from build123d import *

# Parameters (mm, degrees)
F0_W     = 38.1
F0_H     = 762
F0_W_2   = 63.5
F0_H_2   = 57.15
F0_W_3   = 152.4
F0_H_3   = 152.4
F1_DEPTH = 19.05


with BuildPart() as f1:
    # F0 (on Top) → F1 (new body)
    with BuildSketch(Plane.XY):
        Polygon((-669.859934, 405.539142), (-669.859934, -508.860858), (244.540066, -508.860858), (244.540066, 405.539142), (92.140066, 862.739142), (-517.459934, 862.739142), align=None)
        with Locations((-612.709934, -89.760858)):
            Rectangle(F0_W, F0_H, mode=Mode.SUBTRACT)
        with Locations((187.390066, -89.760858)):
            Rectangle(F0_W, F0_H, mode=Mode.SUBTRACT)
        with Locations((-600.009934, 376.964142)):
            Rectangle(F0_W_2, F0_H_2, mode=Mode.SUBTRACT)
        with Locations((-212.659934, 634.139142)):
            Rectangle(F0_W_3, F0_H_3, mode=Mode.SUBTRACT)
        with Locations((174.690066, 376.964142)):
            Rectangle(F0_W_2, F0_H_2, mode=Mode.SUBTRACT)
    extrude(amount=F1_DEPTH)


solid = f1.part
Check sheet for the modelled part. Datum: model origin and axes. Units: mm. Round coordinates to 2 decimals unless told otherwise and drop trailing zeros. Write each loop counter-clockwise with the first axis right and the second up, starting at its lowest first coordinate (ties: lowest second). Pieces come first, ordered by that corner, then holes. Notation, with made-up numbers: (67.5, 18.5) -> (109.5, 18.5) arc R12 cw to (109.5, 29.5) -> close; hole circle Ø6 at (85, 57.5). An arc over 180 degrees is marked (long way). Answer as CSV lines item,"result". Start each with the question number.
1) Material ranges on line 1 (X direction, y = -289.5, z = 4.25); line 2 (X direction, y = 357, z = 2); line 3 (Y direction, x = -166.5, z = 9), recorded low to high. Write a range as from..to.
2) Section check B-B on z = 7. Enter the section's corners in (x, y), and give its area (3 significant figures).
3) Section check D-D on y = 509. Enter the section's corners in (x, z), and give its area (3 significant figures).
4) Section check C-C on x = -197. Enter the section's corners in (y, z), and give its area (3 significant figures).
5) Go/stop test with a flat-tipped pin: P1, Ø5.5, axis at y = 670, z = 11.5, coming from the +X side. Record where the tip stops, or that it passes through.
6) Section check A-A on y = 29.5. Enter the section's corners in (x, z).
Found:
1,line 1,"x = -669.86..-631.76, -593.66..168.34, 206.44..244.54"
1,line 2,"x = -669.86..-631.76, -568.26..142.94, 206.44..244.54"
1,line 3,"y = -508.86..557.94, 710.34..862.74"
2,outline,"(-669.86, -508.86) -> (244.54, -508.86) -> (244.54, 405.54) -> (92.14, 862.74) -> (-517.46, 862.74) -> (-669.86, 405.54) -> close; hole (-631.76, -470.76) -> (-593.66, -470.76) -> (-593.66, 291.24) -> (-631.76, 291.24) -> close; hole (-631.76, 348.39) -> (-568.26, 348.39) -> (-568.26, 405.54) -> (-631.76, 405.54) -> close; hole (-288.86, 557.94) -> (-136.46, 557.94) -> (-136.46, 710.34) -> (-288.86, 710.34) -> close; hole (142.94, 348.39) -> (206.44, 348.39) -> (206.44, 405.54) -> (142.94, 405.54) -> close; hole (168.34, -470.76) -> (206.44, -470.76) -> (206.44, 291.24) -> (168.34, 291.24) -> close"
2,area,"1,100,000 mm^2"
3,outline,"(-635.37, 0) -> (210.05, 0) -> (210.05, 19.05) -> (-635.37, 19.05) -> close"
3,area,"16,100 mm^2"
4,outline,"(-508.86, 0) -> (557.94, 0) -> (557.94, 19.05) -> (-508.86, 19.05) -> close; (710.34, 0) -> (862.74, 0) -> (862.74, 19.05) -> (710.34, 19.05) -> close"
4,area,"23,200 mm^2"
5,P1,"stops at x = 157.3"
6,outline,"(-669.86, 0) -> (-631.76, 0) -> (-631.76, 19.05) -> (-669.86, 19.05) -> close; (-593.66, 0) -> (168.34, 0) -> (168.34, 19.05) -> (-593.66, 19.05) -> close; (206.44, 0) -> (244.54, 0) -> (244.54, 19.05) -> (206.44, 19.05) -> close"
